```python
from build123d import *

# Parameters (mm, degrees)
BASE_FLANGE1_DEPTH      = 25.4
SKETCH6_R               = 5.08
CUT_EXTRUDE1_DEPTH      = 838.117118208
BOSS_EXTRUDE1_OUTLINE_W = 1.905
BOSS_EXTRUDE1_OUTLINE_H = 6.35
BOSS_EXTRUDE1_DEPTH     = 1.905


# Read off the part's stored shape, not the designer's step: Boss-Extrude1
# Sheet-metal steps are written as plain solids
with BuildPart() as part:
    # Sketch1 → Base-Flange1 (new body)
    with BuildSketch(Plane(origin=(0, 836.6125, -836.6125), x_dir=(1, 0, 0), z_dir=(0, -1, 0))):
        with BuildLine():
            Line((432.5239, 836.6125), (432.5239, 853.0209))
            ThreePointArc((432.5239, 853.0209), (433.669581115, 855.786818885), (436.4355, 856.9325))
            Line((436.4355, 856.9325), (449.3895, 856.9325))
            ThreePointArc((449.3895, 856.9325), (452.155418885, 855.786818885), (453.3011, 853.0209))
            Line((453.3011, 853.0209), (453.3011, 836.6125))
            Line((453.3011, 836.6125), (451.3961, 836.6125))
            Line((451.3961, 836.6125), (451.3961, 853.0209))
            ThreePointArc((451.3961, 853.0209), (450.808380467, 854.439780467), (449.3895, 855.0275))
            Line((449.3895, 855.0275), (436.4355, 855.0275))
            ThreePointArc((436.4355, 855.0275), (435.016619533, 854.439780467), (434.4289, 853.0209))
            Line((434.4289, 853.0209), (434.4289, 836.6125))
            Line((434.4289, 836.6125), (432.5239, 836.6125))
        make_face()
    extrude(amount=BASE_FLANGE1_DEPTH)

    # Sketch6 → Cut-Extrude1 (cut, through all)
    with BuildSketch(Plane(origin=(453.3011, 0, 0), x_dir=(0, 0, -1), z_dir=(1, 0, 0))):
        with Locations((-10.16, 821.3725)):
            Circle(SKETCH6_R)
    extrude(amount=-CUT_EXTRUDE1_DEPTH, mode=Mode.SUBTRACT)

    # Boss-Extrude1 outline → Boss-Extrude1 (add)
    with BuildSketch(Plane.XZ.offset(-811.2125)):
        with Locations((452.3486, 9.525)):
            Rectangle(BOSS_EXTRUDE1_OUTLINE_W, BOSS_EXTRUDE1_OUTLINE_H)
        with Locations((433.4764, 9.525)):
            Rectangle(BOSS_EXTRUDE1_OUTLINE_W, BOSS_EXTRUDE1_OUTLINE_H)
    extrude(amount=BOSS_EXTRUDE1_DEPTH)


solid = part.part
```
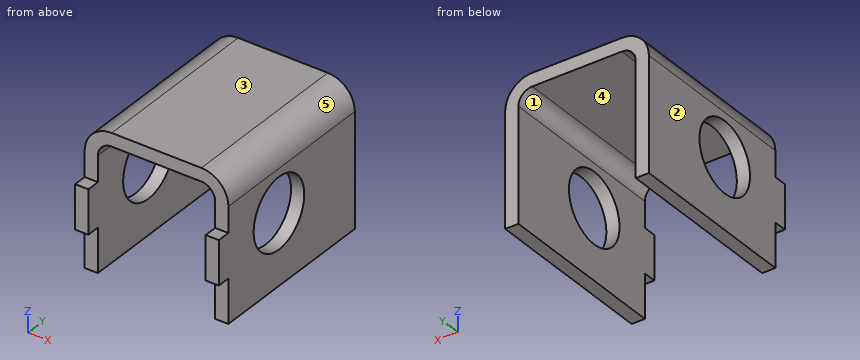
Model file for the job. Use its own axes, mm. Face numbers are marked on the shaded views. A direction names the side the tool comes from. Round coordinates to 2 decimals unless told otherwise and drop trailing zeros. Write each loop counter-clockwise with the first axis right and the second up, starting at its lowest first coordinate (ties: lowest second). Pieces come first, ordered by that corner, then holes. Notation, with made-up numbers: (-15, -23) - (34, -23) arc R20 cw to (34, 5) - close; hole circle Ø5 at (13, 32). An arc over 180 degrees is marked (long way). Use CSV: the item, a comma, the result in double quotes. Start each with the question number.
Item 1: Pin check, flat tips, straight feed: P1, Ø2, axis at x = 433.5, z = 3.5, coming from the -Y side; P2, Ø6.5, axis at x = 440, y = 828, coming from the -Z side (3 decimals); P3, Ø2, axis at x = 452.5, y = 810, coming from the +Z side. Stop position of each tip, or through.
Item 2: Band-saw the part on A-A (z = 3.5). Write the cut outline in (x, y), and give its area (3 significant figures).
Item 3: Drill centre lines: L1, parallel to X at y = 813.5, z = 13.5; L2, parallel to Y at x = 451.9, z = 10.16; L3, parallel to Z at x = 448, y = 811.5 (3 decimals). Where is each one in solid material? Low to high. Write a range as [from, to].
Item 4: Two-plate mould, pull along X, no slides. Class the marked faces 3, 4 and 5: released by +X, released by -X, zero draft, split by the parting line, or undercut.
Item 5: Band-saw the part on D-D (z = 7). Write the cut outline in (x, y), and give its area (3 significant figures).
Item 6: Band-saw the part on B-B (y = 823.75). Write the cut outline in (x, z) (1 decimal).
Item 7: Tool access for the marked faces 1 and 2: list every direction of +Z, -Z, +X, -X, +Y, -Y with a clear straight run to the whole face (end or side of a thin tool).
Item 8: Band-saw the part on C-C (z = 10.16). Write the cut outline in (x, y).
Checked values:
1,P1,"stops at y = 811.21"
1,P2,"stops at z = 18.415"
1,P3,"stops at z = 12.7"
2,outline,"(432.52, 811.21) - (434.43, 811.21) - (434.43, 836.61) - (432.52, 836.61) - close; (451.4, 811.21) - (453.3, 811.21) - (453.3, 836.61) - (451.4, 836.61) - close"
2,area,"96.8 mm²"
3,L1,"x = [432.52, 434.43], [451.4, 453.3]"
3,L2,"y = [809.31, 816.29], [826.45, 836.61]"
3,L3,"z = [18.415, 20.32]"
4,face 3,"zero draft"
4,face 4,"undercut"
4,face 5,"released by +X"
5,outline,"(432.52, 809.31) - (434.43, 809.31) - (434.43, 817.39) - (432.52, 817.39) - close; (432.52, 825.35) - (434.43, 825.35) - (434.43, 836.61) - (432.52, 836.61) - close; (451.4, 809.31) - (453.3, 809.31) - (453.3, 817.39) - (451.4, 817.39) - close; (451.4, 825.35) - (453.3, 825.35) - (453.3, 836.61) - (451.4, 836.61) - close"
5,area,"73.7 mm²"
6,outline,"(432.5, 0) - (434.4, 0) - (434.4, 5.7) - (432.5, 5.7) - close; (432.5, 14.6) - (434.4, 14.6) - (434.4, 16.4) arc R2 cw to (436.4, 18.4) - (449.4, 18.4) arc R2 cw to (451.4, 16.4) - (451.4, 14.6) - (453.3, 14.6) - (453.3, 16.4) arc R3.9 ccw to (449.4, 20.3) - (436.4, 20.3) arc R3.9 ccw to (432.5, 16.4) - close; (451.4, 0) - (453.3, 0) - (453.3, 5.7) - (451.4, 5.7) - close"
7,face 1,"-Z, +Y, -Y"
7,face 2,"+Z, -Z, -X, +Y, -Y"
8,outline,"(432.52, 809.31) - (434.43, 809.31) - (434.43, 816.29) - (432.52, 816.29) - close; (432.52, 826.45) - (434.43, 826.45) - (434.43, 836.61) - (432.52, 836.61) - close; (451.4, 809.31) - (453.3, 809.31) - (453.3, 816.29) - (451.4, 816.29) - close; (451.4, 826.45) - (453.3, 826.45) - (453.3, 836.61) - (451.4, 836.61) - close"
